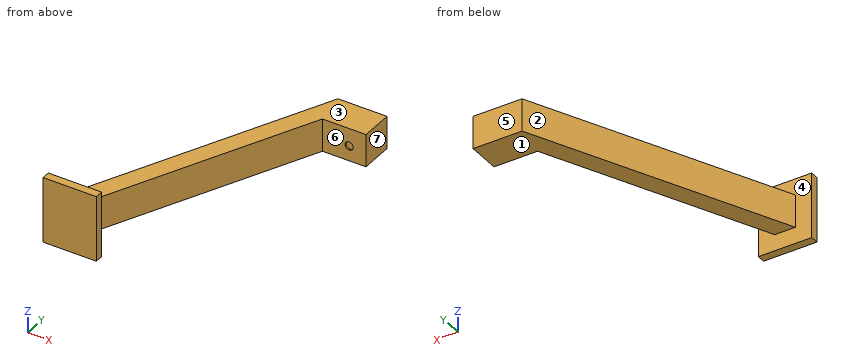
from build123d import *

# Parameters (mm, degrees)
BOSS_EXTRUDE1_DEPTH = 20
SKETCH2_W           = 32.657953652
SKETCH2_H           = 40
BOSS_EXTRUDE2_DEPTH = 5
SKETCH3_R           = 2.5
CUT_EXTRUDE1_DEPTH  = 1


with BuildPart() as part:
    # Sketch1 → Boss-Extrude1 (new body)
    with BuildSketch(Plane.XY):
        Polygon((-11.668199512, -10), (-72.614610432, -140.7), (-85.272564084, -140.7), (-15, 10), (15, 10), (15, -10), align=None)
    extrude(amount=BOSS_EXTRUDE1_DEPTH)

    # Sketch2 → Boss-Extrude2 (add)
    with BuildSketch(Plane.XZ.offset(140.7)):
        with Locations((-78.943587258, 10)):
            Rectangle(SKETCH2_W, SKETCH2_H)
    extrude(amount=BOSS_EXTRUDE2_DEPTH)

    # Sketch3 → Cut-Extrude1 (cut)
    with BuildSketch(Plane.XZ.offset(10)):
        with Locations((4.736957345, 9.180800469)):
            Circle(SKETCH3_R)
    extrude(amount=-CUT_EXTRUDE1_DEPTH, mode=Mode.SUBTRACT)


solid = part.part
The model under review builds one solid part; all positions refer to its coordinate system, in mm. Face numbers are marked on the shaded views. A direction names the side the tool comes from. Round coordinates to 2 decimals unless told otherwise and drop trailing zeros. Write each loop counter-clockwise with the first axis right and the second up, starting at its lowest first coordinate (ties: lowest second). Pieces come first, ordered by that corner, then holes. Notation, with made-up numbers: M 81.5,9.5 L 117.5,9.5 A23 ccw 117.5,40.5 Z; hole C -32,71 d4. An arc over 180 degrees is marked long. Use a Markdown table: item, result. Add a question column.
Q1. Insertion check: pin 1 (3 mm diameter, centred on x = -56.5, z = 5.5, fed in from -Y); pin 2 (6 mm diameter, centred on x = 4.74, z = 9.18, fed in from -Y); pin 3 (2.5 mm diameter, centred on y = -143, z = 1, fed in from +X). Each pin has a flat end and moves straight along its axis. Give the tip position at first contact, or say it passes through.
Q2. Machinability: for the marked faces 1, 2 and 3, which of the approach directions +Z, -Z, +X, -X, +Y, -Y give a long, thin tool a straight path to every point of the face, cutting with its end or side? Answer none if there is none.
Q3. We need section A-A, the plane z = 2. State the section outline as (x, y) points.
Q4. The part is to be moulded in two halves that separate along Y. For the marked faces 4, 5, 6 and 7, say which applies: pulls with the +Y half, pulls with the -Y half, needs draft (parallel to the pull), parting line crosses it, or undercut.
Q5. We need section C-C, the plane y = -87. State the section outline as (x, z) points, plus the area to 3 significant figures.
Q6. To check wall thickness, follow line 1 (Y direction, x = 9, z = 14.5); line 2 (X direction, y = -51.5, z = 6.5); line 3 (Y direction, x = -45, z = 18.5). State the ranges of each line that lie inside material, in increasing order.
Q7. We need section B-B, the plane x = -3. State the section outline as (y, z) points.
Findings below:
| question | item | result |
|---|---|---|
| 1 | pin 1 | stops at y = -109.36 |
| 1 | pin 2 | stops at y = -10 |
| 1 | pin 3 | stops at x = -62.61 |
| 2 | face 1 | -Z, +X, -X, +Y |
| 2 | face 2 | +Z, -Z, -X, +Y |
| 2 | face 3 | +Z, +X, -X, +Y |
| 3 | outline | M -95.27,-145.7 L -62.61,-145.7 L -62.61,-140.7 L -72.61,-140.7 L -11.67,-10 L 15,-10 L 15,10 L -15,10 L -85.27,-140.7 L -95.27,-140.7 Z |
| 4 | face 4 | undercut |
| 4 | face 5 | pulls with the +Y half |
| 4 | face 6 | pulls with the -Y half |
| 4 | face 7 | needs draft |
| 5 | outline | M -60.23,0 L -47.57,0 L -47.57,20 L -60.23,20 Z |
| 5 | area | 253 mm² |
| 6 | line 1 | y = -10 to 10 |
| 6 | line 2 | x = -43.68 to -31.02 |
| 6 | line 3 | y = -81.48 to -54.34 |
| 7 | outline | M -10,0 L 10,0 L 10,20 L -10,20 Z |
